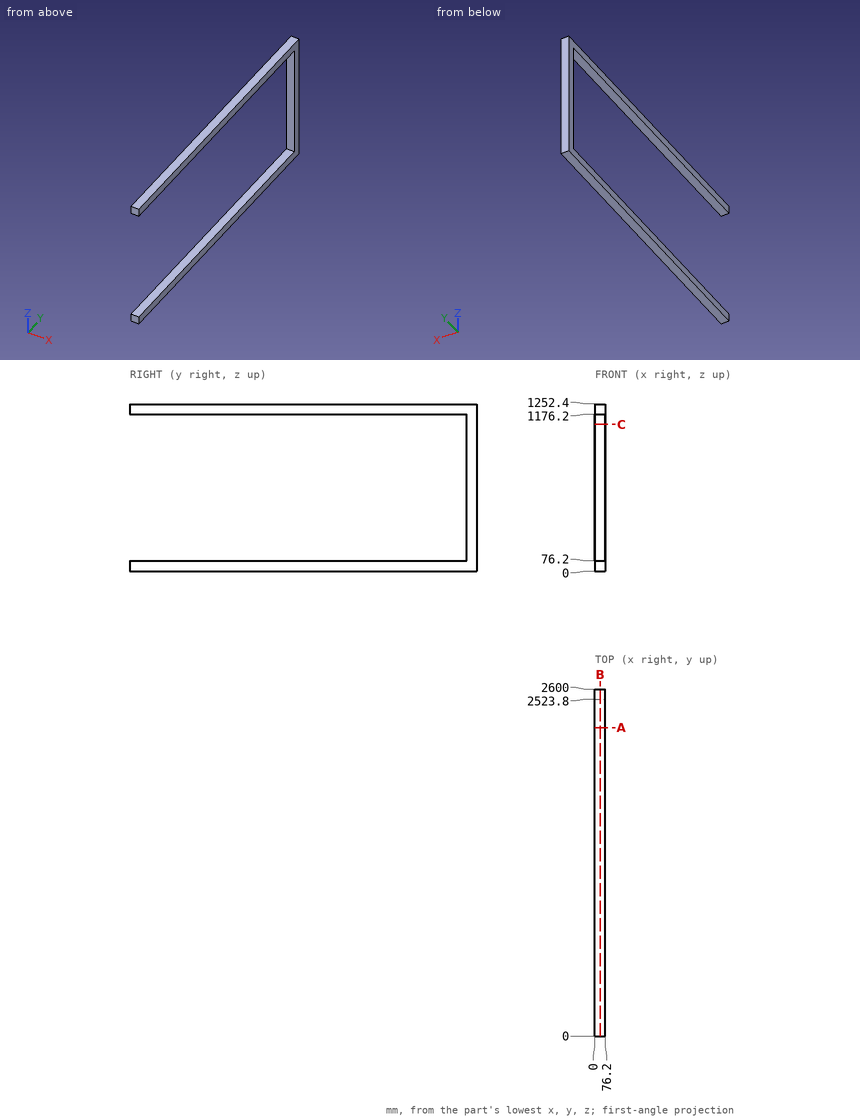
Here's the drawing with two shaded views (mm, measured from the low corner). I have some questions. Give positions to 0.01 mm unless a question says otherwise; leave off trailing zeros. Loops run counter-clockwise (first coordinate to the right, second up) from the corner with the lowest first, then second, coordinate; pieces in that order, holes last. Notation, with made-up numbers: (-24.75, -5.75) -> (25.25, -5.75) arc R26 ccw to (25.25, 18.25) -> close; hole circle Ø10 at (-29, 54). An arc over 180 degrees is marked (long way). One line per item, written item: value.
Q1. If I drill on line 1 along Z through (x, y) = (56, 1132.5); line 2 along Y through (x, z) = (49.5, 598), over which ranges is the centre line in solid material (lowest first)?
Answers follow:
line 1: 0 to 76.2, 1176.2 to 1252.4
line 2: 2523.8 to 2600
Q2. Suppose I cut it at A-A on y = 2310.5. Please give me the cut outline in (x, z), then the cut area to 3 significant figures.
Answers follow:
outline: (0, 0) -> (76.2, 0) -> (76.2, 76.2) -> (0, 76.2) -> close; (0, 1176.2) -> (76.2, 1176.2) -> (76.2, 1252.4) -> (0, 1252.4) -> close
area: 11,600 mm^2
Q3. Suppose I cut it at C-C on z = 1099. Please give me the cut outline in (x, y).
Answers follow:
outline: (0, 2523.8) -> (76.2, 2523.8) -> (76.2, 2600) -> (0, 2600) -> close
Q4. Suppose I cut it at B-B on x = 39.5. Please give me the cut outline in (y, z).
Answers follow:
outline: (0, 0) -> (2600, 0) -> (2600, 1252.4) -> (0, 1252.4) -> (0, 1176.2) -> (2523.8, 1176.2) -> (2523.8, 76.2) -> (0, 76.2) -> close
